Could you check a few things on this model? Use its own coordinates, in mm. A direction names the side the tool comes from. Give positions to 0.01 mm unless a question says otherwise; leave off trailing zeros. Loops run counter-clockwise (first coordinate to the right, second up) from the corner with the lowest first, then second, coordinate; pieces in that order, holes last. Notation, with made-up numbers: M -6.75,-11 L 52.25,-11 A23 cw 52.25,9 Z; hole C -12.75,-13.75 d9. An arc over 180 degrees is marked long. Answer in a Markdown table with one row per item. Add a question column.
1. I need wall thicknesses on line 1 along Z through (x, y) = (8, 23.7); line 2 along Z through (x, y) = (-8, 24.8); line 3 along X through (y, z) = (-24.3, 46). Which ranges of each line are inside material? Lowest first, please. Write a range as from..to.
2. If we section it at B-B on x = -8: Count the separate pieces of the cut face and the enclosed holes in it, then the cut area to 3 significant figures.
3. If we section it at A-A on z = 46: List the corners of the cut face in (x, y) for me, then the cut area to 3 significant figures.
4. Which directions (+Z, -Z, +X, -X, +Y, -Y) give clear straight access to the entire face, cutting with the end or side of a thin tool? Please do faces 4 (the flat face through (-10.5, 0, 25)), 5 (the flat face through (6.5, 24, 17)), 6 (the flat face through (-7, 24.5, 41)), 7 (the cylindrical face through (-8.07, 23.99, 44.5)).
5. I'm going to push flat-ended pins straight in: pin 1 Ø3 at (x, z) = (-4, 34) entering from +Y; pin 2 Ø2.5 at (x, z) = (-8, 40) entering from +Y. Where does each tip first touch, or does it pass through?
6. If we section it at C-C on y = 10: List the corners of the cut face in (x, z) for me.
7. If we section it at D-D on z = 10.5: List the corners of the cut face in (x, y) for me.
8. Thinking about a two-plate mould opening in X: for faces 1 (the flat face through (-11, 2, 50)), 2 (the flat face through (-12.5, 0, 25)), 3 (the cylindrical face through (8.9, 24, 44.8)), which applies, released by +X, released by -X, zero draft, split by the parting line, or undercut?
Autodesk Inventor part; units mm, degrees
ref_plane "YZ Plane" through (0, 0, 0) normal (1, 0, 0) x (0, 1, 0)
ref_plane "XZ Plane" through (0, 0, 0) normal (0, 1, 0) x (-1, 0, 0)
ref_plane "XY Plane" through (0, 0, 0) normal (0, 0, 1) x (1, 0, 0)
sketch "スケッチ1" plane through (0, 0, 0) normal (0, 0, 1) x (1, 0, 0)
  line L0 (-12.5, 25) -> (12.5, 25)
  line L1 (12.5, 25) -> (12.5, -25)
  line L2 (12.5, -25) -> (-12.5, -25)
  line L3 (-12.5, -25) -> (-12.5, 25)
  line L4 (-10.5, 23) -> (10.5, 23)
  line L5 (10.5, 23) -> (10.5, -23)
  line L6 (10.5, -23) -> (-10.5, -23)
  line L7 (-10.5, -23) -> (-10.5, 23)
  point P0 (0, 0)
  dimension "d0" = 25
  dimension "d1" = 50
  dimension "d2" = 46
  dimension "d3" = 21
  dimension "d4" = 25
  dimension "d5" = 23
  dimension "d6" = 10.5
  dimension "d7" = 12.5
extrude "押し出し1" add sketch "スケッチ1" along normal blind 50
sketch "スケッチ2" plane through (-12.5, 25, 0) normal (0, 1, 0) x (1, 0, 0)
  line L0 (0, 0) -> (25, 0)
  line L1 (0, 0) -> (0, -50)
  arc A0 (6, -33.5) -> (19, -33.5) centre (12.5, -33.5) ccw
  line L2 (6, -33.5) -> (6, 0)
  line L3 (19, -33.5) -> (19, 0)
  point P0 (12.5, 0)
  dimension "d10" = 13
  dimension "d11" = 33.5
  dimension "d12" = 12.5
extrude "押し出し2" cut sketch "スケッチ2" against normal blind 2
sketch "スケッチ3" plane through (-12.5, 25, 50) normal (0, 1, 0) x (1, 0, 0)
  arc A0 (6, 16.5) -> (19, 16.5) centre (12.5, 16.5) ccw
  circle A1 centre (4.5, 10) radius 1
  circle A2 centre (4.5, 46) radius 1
  circle A3 centre (20.5, 46) radius 1
  circle A4 centre (20.5, 10) radius 1
  point P0 (12.5, 50)
  dimension "d15" = 6.5
  dimension "d16" = 6.5
  dimension "d17" = 2
  dimension "d18" = 8
  dimension "d19" = 8
  dimension "d20" = 8
  dimension "d21" = 8
  dimension "d22" = 29.5
  dimension "d23" = 29.5
hole "穴1" at (-8, 25, 4) at (8, 25, 4) at (8, 25, 40) at (-8, 25, 40) direction (0, -1, 0) diameter 2 depth 2 tip angle 118 counterbore diameter 4 counterbore depth 0.5
sketch "スケッチ4" plane through (-12.5, -25, 0) normal (0, -1, 0) x (1, 0, 0)
  line L0 (25, 0) -> (0, 0)
  line L1 (25, 0) -> (25, 50)
  circle A0 centre (12.5, 10.5) radius 2
  point P0 (12.5, 0)
  dimension "d31" = 4
  dimension "d32" = 12.5
  dimension "d33" = 10.5
hole "穴2" at (0, -25, 10.5) direction (0, 1, 0) diameter 4 end through all
sketch "スケッチ5" plane through (-12.5, 25, 50) normal (0, 1, 0) x (1, 0, 0)
  line L0 (0, 0) -> (25, 0)
  arc A0 (6, 16.5) -> (19, 16.5) centre (12.5, 16.5) ccw
  circle A1 centre (20.5, 4) radius 1.5
  circle A2 centre (4.5, 4) radius 1.5
  point P0 (12.5, 50)
  dimension "d43" = 4
  dimension "d44" = 4
  dimension "d46" = 8
  dimension "d47" = 8
  dimension "d57" = 3
hole "穴4" at (-8, 25, 46) at (8, 25, 46) direction (0, -1, 0) diameter 3 end through all
thread "ねじ1"
thread "ねじ2"
thread "ねじ3"
thread "ねじ4"
properties part number "14" material "アルミニウム 6061"
Results:
| question | item | result |
|---|---|---|
| 1 | line 1 | 0..3, 5..39, 41..44.5, 47.5..50 |
| 1 | line 2 | 0..2, 6..38, 42..44.5, 47.5..50 |
| 1 | line 3 | -12.5..-9.5, -6.5..6.5, 9.5..12.5 |
| 2 | separate pieces | 6 |
| 2 | enclosed holes | 0 |
| 2 | area | 178 mm2 |
| 3 | outline | M -12.5,-25 L -9.5,-25 L -9.5,-23 L -10.5,-23 L -10.5,23 L -9.5,23 L -9.5,25 L -12.5,25 Z; M -6.5,-25 L 6.5,-25 L 6.5,-23 L -6.5,-23 Z; M -6.5,23 L 6.5,23 L 6.5,25 L -6.5,25 Z; M 9.5,-25 L 12.5,-25 L 12.5,25 L 9.5,25 L 9.5,23 L 10.5,23 L 10.5,-23 L 9.5,-23 Z |
| 3 | area | 260 mm2 |
| 4 | face 4 | +Z, -Z |
| 4 | face 5 | -Z, +Y |
| 4 | face 6 | +Y |
| 4 | face 7 | +Y, -Y |
| 5 | pin 1 | y = -23 |
| 5 | pin 2 | y = 24.5 |
| 6 | outline | M -12.5,0 L -10.5,0 L -10.5,50 L -12.5,50 Z; M 10.5,0 L 12.5,0 L 12.5,50 L 10.5,50 Z |
| 7 | outline | M -12.5,-25 L -2,-25 L -2,-23 L -10.5,-23 L -10.5,23 L -6.5,23 L -6.5,25 L -12.5,25 Z; M 2,-25 L 12.5,-25 L 12.5,25 L 6.5,25 L 6.5,23 L 10.5,23 L 10.5,-23 L 2,-23 Z |
| 8 | face 1 | zero draft |
| 8 | face 2 | released by -X |
| 8 | face 3 | undercut |
